```python
from build123d import *

# Parameters (mm, degrees)
SKETCH_1_W           = 20
SKETCH_1_H           = 40
EXTRUDE_1_DEPTH      = 37
SKETCH_2_R           = 0.75
CUT_EXTRUDE_10_DEPTH = 2
SKETCH_3_R           = 10
EXTRUDE_3_DEPTH      = 2
SKETCH_4_R           = 2.167388434
EXTRUDE_4_DEPTH      = 3
SKETCH_5_W           = 20
SKETCH_5_H           = 3
EXTRUDE_5_DEPTH      = 5
SKETCH_6_R           = 2.5
CUT_EXTRUDE_13_DEPTH = 3
SKETCH_9_W           = 20
SKETCH_9_H           = 3
EXTRUDE_7_DEPTH      = 5
SKETCH_10_R          = 2.5
CUT_EXTRUDE_14_DEPTH = 3


with BuildPart() as part:
    # 草图1 → 凸台-拉伸1 (new body)
    with BuildSketch(Plane(origin=(0, 0, 0), x_dir=(1, 0, 0), z_dir=(0, 1, 0))):
        Rectangle(SKETCH_1_W, SKETCH_1_H)
    extrude(amount=EXTRUDE_1_DEPTH)

    # 草图2 → 切除-拉伸10 (cut)
    with BuildSketch(Plane(origin=(0, 0, 0), x_dir=(1, 0, 0), z_dir=(0, 1, 0))):
        with Locations((-9, 19)):
            Circle(SKETCH_2_R)
        with Locations((9, 19)):
            Circle(SKETCH_2_R)
        with Locations((-9, -19)):
            Circle(SKETCH_2_R)
        with Locations((9, -19)):
            Circle(SKETCH_2_R)
    extrude(amount=CUT_EXTRUDE_10_DEPTH, mode=Mode.SUBTRACT)

    # 草图3 → 凸台-拉伸3 (add)
    with BuildSketch(Plane(origin=(0, 37, 0), x_dir=(1, 0, 0), z_dir=(0, 1, 0))):
        with Locations((0, -10)):
            Circle(SKETCH_3_R)
    extrude(amount=EXTRUDE_3_DEPTH)

    # 草图4 → 凸台-拉伸4 (add)
    with BuildSketch(Plane(origin=(0, 39, 0), x_dir=(1, 0, 0), z_dir=(0, 1, 0))):
        with Locations((0, -10)):
            Circle(SKETCH_4_R)
    extrude(amount=EXTRUDE_4_DEPTH)

    # 草图5 → 凸台-拉伸5 (add)
    with BuildSketch(Plane.XY.offset(20)):
        with Locations((0, 30.61035469)):
            Rectangle(SKETCH_5_W, SKETCH_5_H)
    extrude(amount=EXTRUDE_5_DEPTH)

    # 草图6 → 切除-拉伸13 (cut)
    with BuildSketch(Plane(origin=(0, 32.11035469, 0), x_dir=(1, 0, 0), z_dir=(0, 1, 0))):
        with Locations((-6, -23.644142826)):
            Circle(SKETCH_6_R)
        with Locations((6, -23.644142826)):
            Circle(SKETCH_6_R)
    extrude(amount=-CUT_EXTRUDE_13_DEPTH, mode=Mode.SUBTRACT)

    # 草图9 → 凸台-拉伸7 (add)
    with BuildSketch(Plane(origin=(0, 0, -20), x_dir=(-1, 0, 0), z_dir=(0, 0, -1))):
        with Locations((0, 30.5)):
            Rectangle(SKETCH_9_W, SKETCH_9_H)
    extrude(amount=EXTRUDE_7_DEPTH)

    # 草图10 → 切除-拉伸14 (cut)
    with BuildSketch(Plane(origin=(0, 32, 0), x_dir=(1, 0, 0), z_dir=(0, 1, 0))):
        with Locations((-6, 24)):
            Circle(SKETCH_10_R)
        with Locations((6, 24)):
            Circle(SKETCH_10_R)
    extrude(amount=-CUT_EXTRUDE_14_DEPTH, mode=Mode.SUBTRACT)


solid = part.part
```
Check sheet for the modelled part. Datum: model origin and axes. Units: mm. A direction names the side the tool comes from. Round coordinates to 2 decimals unless told otherwise and drop trailing zeros. Write each loop counter-clockwise with the first axis right and the second up, starting at its lowest first coordinate (ties: lowest second). Pieces come first, ordered by that corner, then holes. Notation, with made-up numbers: (88.5, 62.5) -> (92.5, 62.5) arc R31 ccw to (92.5, 96.5) -> close; hole circle Ø6 at (-19, 46). An arc over 180 degrees is marked (long way). Put each result on its own line as item: value.
(1) Mould release check, pull along X, two halves, no side actions. Record for faces 1 (the face through (9, 2, 19)), 2 (the face through (0, 29, -22)), 3 (the face through (-10, 18, 0)), 4 (the face through (10, 18, 0)): released by +X, released by -X, zero draft, split by the parting line, or undercut.
Values found:
face 1: undercut
face 2: zero draft
face 3: released by -X
face 4: released by +X
(2) Sectioned sample at A-A (z = -24). Enter the section's corners in (x, y).
Values found:
outline: (-10, 29) -> (-8.5, 29) -> (-8.5, 32) -> (-10, 32) -> close; (-3.5, 29) -> (3.5, 29) -> (3.5, 32) -> (-3.5, 32) -> close; (8.5, 29) -> (10, 29) -> (10, 32) -> (8.5, 32) -> close
(3) Sectioned sample at B-B (x = 6). Enter the section's corners in (y, z).
Values found:
outline: (0, -20) -> (29, -20) -> (29, -21.5) -> (32, -21.5) -> (32, -20) -> (37, -20) -> (37, 2) -> (39, 2) -> (39, 18) -> (37, 18) -> (37, 20) -> (32.11, 20) -> (32.11, 21.14) -> (29.11, 21.14) -> (29.11, 20) -> (0, 20) -> close
(4) Tool access check on faces 5 (the face through (8.405, 0.986, 19.456)), 6 (the face through (0, 14, -20)), 7 (the face through (0, 34, -20)), 8 (the face through (-8, 37, 18)). Record the directions out of +Z, -Z, +X, -X, +Y, -Y that give a thin tool (end or side, any length) a straight path to the whole face; none if there is none.
Values found:
face 5: -Y
face 6: -Z, +X, -X, -Y
face 7: -Z, +X, -X, +Y
face 8: +Z, -X, +Y
(5) Sectioned sample at C-C (z = -3). Enter the section's corners in (x, y), plus the area to 3 significant figures.
Values found:
outline: (-10, 0) -> (10, 0) -> (10, 37) -> (-10, 37) -> close
area: 740 mm^2
(6) Material ranges on line 1 (Z direction, x = 9, y = 1.65); line 2 (X direction, y = 30.3, z = -24); line 3 (X direction, y = 1.1, z = 19), recorded low to high.
Values found:
line 1: z = -20 to -19.75, -18.25 to 18.25, 19.75 to 20
line 2: x = -10 to -8.5, -3.5 to 3.5, 8.5 to 10
line 3: x = -10 to -9.75, -8.25 to 8.25, 9.75 to 10
(7) Go/stop test with flat-tipped pins: pin 1 Ø10 at (x, z) = (0.5, -18.5) entering from +Y; pin 2 Ø2 at (x, y) = (6.5, 28) entering from +Z; pin 3 Ø1.5 at (x, z) = (2.5, -23) entering from -Y. Record where each tip stops, or that it passes through.
Values found:
pin 1: stops at y = 37
pin 2: stops at z = 20
pin 3: stops at y = 29
(8) Sectioned sample at D-D (y = 19). Enter the section's corners in (x, z), plus the area to 3 significant figures.
Values found:
outline: (-10, -20) -> (10, -20) -> (10, 20) -> (-10, 20) -> close
area: 800 mm^2
